from build123d import *

# Parameters (mm, degrees)
F0_R     = 50
F0_R_2   = 30
F1_DEPTH = 200
F2_W     = 40
F2_H     = 80
F3_DEPTH = 4950
F4_W     = 40
F4_H     = 80
F5_DEPTH = 2839


with BuildPart() as f1:
    # F0 (on Top) → F1 (new body)
    with BuildSketch(Plane.XY):
        Circle(F0_R)
        Circle(F0_R_2, mode=Mode.SUBTRACT)
    extrude(amount=F1_DEPTH)

    # F2 (on Front) → F3 (cut, symmetric)
    with BuildSketch(Plane.XZ):
        Rectangle(F2_W, F2_H)
    extrude(amount=F3_DEPTH, both=True, mode=Mode.SUBTRACT)

    # F4 (on Right) → F5 (cut, symmetric)
    with BuildSketch(Plane.YZ):
        Rectangle(F4_W, F4_H)
    extrude(amount=F5_DEPTH, both=True, mode=Mode.SUBTRACT)


solid = f1.part
Read the model definition and answer for the solid it produces. Units are mm, in the model's axes. A direction names the side the tool comes from. Coordinates: 2 decimals unless noted, no trailing zeros. Write each loop counter-clockwise with the first axis right and the second up, starting at its lowest first coordinate (ties: lowest second). Pieces come first, ordered by that corner, then holes. Notation, with made-up numbers: (53, -35.5) -> (104, -35.5) arc R12 ccw to (104, -24.5) -> close; hole circle Ø11 at (-9, 17.25). An arc over 180 degrees is marked (long way). Return JSON: item names as keys, results as strings.
(1) The part is cut by section B-B on y = 0. Give the vertices of the cut face in (x, z).
Answers below:
{"outline": "(-50, 40) -> (-30, 40) -> (-30, 200) -> (-50, 200) -> close; (30, 40) -> (50, 40) -> (50, 200) -> (30, 200) -> close"}
(2) Consider line 1 along Y through (x, z) = (0, 43.5); line 2 along Y through (x, z) = (-9.5, 133.5); line 3 along Z through (x, y) = (33, 19.5). Determine where each line is inside the solid, lowest interval first. Write a range as from..to.
Answers below:
{"line 1": "-50..-30, 30..50", "line 2": "-49.09..-28.46, 28.46..49.09", "line 3": "40..200"}
(3) Each of these flat-tipped pins is pushed along its axis until it touches: P1, Ø8, axis at x = 39.5, z = 52.5, coming from the -Y side; P2, Ø19, axis at y = 35.5, z = 23.5, coming from the -X side; P3, Ø8, axis at y = 5.5, z = 119.5, coming from the -X side. Where does it stop, or does it pass through?
Answers below:
{"P1": "y = -35.21", "P2": "x = -42.71", "P3": "x = -49.98"}
(4) The part is cut by section D-D on y = -39. Give the vertices of the cut face in (x, z).
Answers below:
{"outline": "(-31.29, 0) -> (-20, 0) -> (-20, 40) -> (20, 40) -> (20, 0) -> (31.29, 0) -> (31.29, 200) -> (-31.29, 200) -> close"}
(5) Which of the six approach directions +Z, -Z, +X, -X, +Y, -Y give full straight-line access (tool end or side, diameter ignored) to faces 1 (the flat face through (22, -22, 200)), 2 (the flat face through (-20, 34, 20)), 3 (the flat face through (-34, -20, 20))?
Answers below:
{"face 1": "+Z, +X, -X, +Y, -Y", "face 2": "-Z, +Y, -Y", "face 3": "-Z, +X, -X"}
(6) For a pull along X with two mould halves and no side action, classify faces 4 (the cylindrical face through (-49.95, 2.2, 98.6)), 5 (the flat face through (20, -34, 20)), 6 (the flat face through (34, -20, 20)) as pulls with the +X half, pulls with the -X half, needs draft (parallel to the pull), parting line crosses it, or undercut.
Answers below:
{"face 4": "parting line crosses it", "face 5": "undercut", "face 6": "needs draft"}
(7) The part is cut by section A-A on z = 20. Give the vertices of the cut face in (x, y).
Answers below:
{"outline": "(-45.83, -20) arc R50 ccw to (-20, -45.83) -> (-20, -22.36) arc R30 cw to (-22.36, -20) -> close; (-45.83, 20) -> (-22.36, 20) arc R30 cw to (-20, 22.36) -> (-20, 45.83) arc R50 ccw to start; (20, -45.83) arc R50 ccw to (45.83, -20) -> (22.36, -20) arc R30 cw to (20, -22.36) -> close; (20, 22.36) arc R30 cw to (22.36, 20) -> (45.83, 20) arc R50 ccw to (20, 45.83) -> close"}
